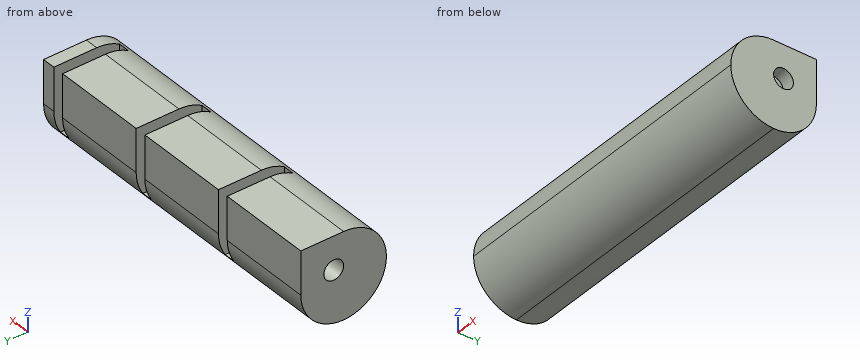
```python
from build123d import *

# Parameters (mm, degrees)
F0_W     = 50
F0_H     = 13
F1_DEPTH = 13
F2_R     = 1.5
F3_DEPTH = 50.001
F4_R     = 6.49999
F5_W     = 1.7
F5_H     = 10
F6_DEPTH = 10


# Not quite as in the source:
# - a fillet or chamfer is up to 0.001 mm smaller than in the source, because OpenCascade refuses the exact size
# - a feature names something its author has since deleted; it is built from what else it names


with BuildPart() as f1:
    # F0 (on Top) → F1 (new body)
    with BuildSketch(Plane.XY):
        with Locations((0.8589621633, -0.6415863931)):
            Rectangle(F0_W, F0_H)
    extrude(amount=F1_DEPTH)

    # F2 (on face) → F3 (cut, through all)
    with BuildSketch(Plane.YZ.offset(25.8589621633)):
        with Locations((0.8584136069, 8)):
            Circle(F2_R)
    extrude(amount=-F3_DEPTH, mode=Mode.SUBTRACT)

    # F4 (radius 6.5 in the source; OpenCascade refuses exactly that, so slightly less here)
    f4_edges = [f1.edges().sort_by_distance(p)[0] for p in [
        (0.858962, -7.141586, 13),
        (0.858962, -7.141586, 0),
        (0.858962, 5.858414, 0),
    ]]
    fillet(f4_edges, radius=F4_R)

    # F5 (on face) → F6 (cut)
    with BuildSketch(Plane.XY.offset(13)):
        with Locations((23.0089621633, 0.8584136069)):
            Rectangle(F5_W, F5_H)
        with Locations((7.0089621633, 0.8584136069)):
            Rectangle(F5_W, F5_H)
        with Locations((-8.9910378367, 0.8584136069)):
            Rectangle(F5_W, F5_H)
    extrude(amount=-F6_DEPTH, mode=Mode.SUBTRACT)


solid = f1.part
```
The model under review builds one solid part; all positions refer to its coordinate system, in mm. Round coordinates to 2 decimals unless told otherwise and drop trailing zeros. Loops run counter-clockwise (first coordinate to the right, second up) from the corner with the lowest first, then second, coordinate; pieces in that order, holes last. Notation, with made-up numbers: M -19.5,32.25 L -3.5,32.25 A32 ccw -3.5,62.25 Z; hole C 41.25,-15 d2. An arc over 180 degrees is marked long. Answer as a JSON object with one key per item and string values.
(1) Take a section at D-D on z = 3.75. Give the boundary of the cut face in (x, y), and give its area (3 significant figures).
Resolved:
{"outline": "M -24.14,-6.53 L 25.86,-6.53 L 25.86,5.25 L 23.86,5.25 L 23.86,-4.14 L 22.16,-4.14 L 22.16,5.25 L 7.86,5.25 L 7.86,-4.14 L 6.16,-4.14 L 6.16,5.25 L -8.14,5.25 L -8.14,-4.14 L -9.84,-4.14 L -9.84,5.25 L -24.14,5.25 Z", "area": "541 mm²"}
(2) To check wall thickness, follow line 1 along X through (y, z) = (2, 5.25); line 2 along Z through (x, y) = (-19.5, 1.25); line 3 along Z through (x, y) = (6, 2). State the ranges of each line that lie inside material, in increasing order.
Resolved:
{"line 1": "-24.14 to -9.84, -8.14 to 6.16, 7.86 to 22.16, 23.86 to 25.86", "line 2": "0.28 to 6.55, 9.45 to 13", "line 3": "0.56 to 7.03, 8.97 to 13"}
(3) Clearance check with flat-ended pins moving along their axes: P1, Ø1, axis at x = -18, z = 3.5, coming from the +Y side; P2, Ø0.8, axis at x = -8.5, z = 5.5, coming from the +Y side; P3, Ø0.5, axis at x = 7.5, y = 2.5, coming from the +Z side; P4, Ø2.5, axis at y = 0.86, z = 8, coming from the -X side. State where each tip first meets the part, or that it passes through.
Resolved:
{"P1": "y = 5.36", "P2": "y = 5.81", "P3": "z = 3", "P4": "through"}
(4) Take a section at B-B on y = 0.75. Count the separate pieces of the cut face and the enclosed holes in it, and give its area (3 significant figures).
Resolved:
{"separate pieces": "5", "enclosed holes": "0", "area": "457 mm²"}
